Here's how the part is built. I have some questions about the finished solid (model axes, mm). Face numbers are marked on the shaded views. A direction names the side the tool comes from. Round coordinates to 2 decimals unless told otherwise and drop trailing zeros. Loops run counter-clockwise (first coordinate to the right, second up) from the corner with the lowest first, then second, coordinate; pieces in that order, holes last. Notation, with made-up numbers: M -36.5,76.5 L -17.5,76.5 A12 ccw -17.5,83.5 Z; hole C -9.75,52.25 d11. An arc over 180 degrees is marked long. Answer as CSV lines item,"result".
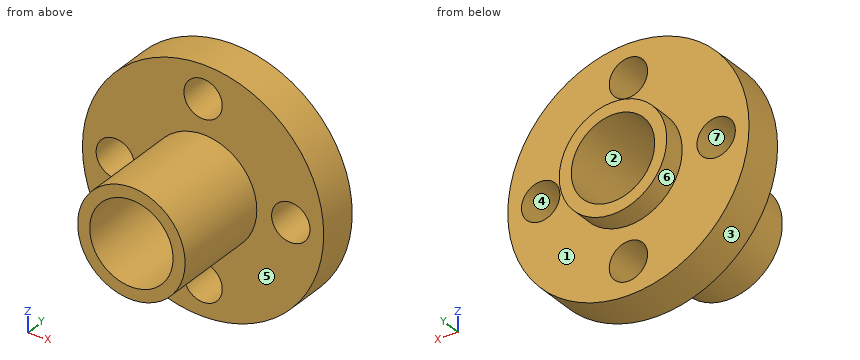
Autodesk Inventor part; units mm, degrees
ref_plane "YZ Plane" through (0, 0, 0) normal (1, 0, 0) x (0, 1, 0)
ref_plane "XZ Plane" through (0, 0, 0) normal (0, 1, 0) x (-1, 0, 0)
ref_plane "XY Plane" through (0, 0, 0) normal (0, 0, 1) x (1, 0, 0)
sketch "Sketch1" plane through (0, 0, 0) normal (0, 0, 1) x (1, 0, 0)
  line L0 (3.8, 0) -> (3.8, 15)
  line L1 (3.8, 15) -> (4.9, 15)
  line L2 (4.9, 15) -> (4.9, 13)
  line L3 (4.9, 13) -> (11, 13)
  line L4 (11, 13) -> (11, 9.3)
  line L5 (11, 9.3) -> (4.9, 9.3)
  line L6 (4.9, 9.3) -> (4.9, 0)
  line L7 (4.9, 0) -> (3.8, 0)
  line L8 (-2.2, 0) -> (13.2, 0)
  line L9 (0, -3) -> (0, 18)
  point P0 (0, 0)
  point P1 (4.35, 0)
  point P2 (4.35, 15)
  point P3 (11, 11.15)
  dimension "d0" = 3.7
  dimension "d1" = 15
  dimension "d2" = 2
  dimension "d3" = 11
  dimension "d4" = 6.1
  dimension "d5" = 3.8
revolve "Revolution1" add sketch "Sketch1" angle 360 about axis through (0, -10, 0) along (0, 1, 0)
sketch "Sketch2" plane through (0, 13, 0) normal (0, 1, 0) x (1, 0, 0)
  circle A0 centre (0, 8) radius 1.75
  point P0 (0, 0)
  dimension "d7" = 3.5
  dimension "d8" = 8
extrude "Extrusion1" cut sketch "Sketch2" against normal up to surface (3.7 mm away)
pattern_circular "Circular Pattern1" count 4 over 360 about axis through (0, 11.15, 0) along (0, 1, 0) of "Extrusion1"
properties part number "Lead nut"
1. I want a section at D-D, the plane y = 8. Please give me the cut outline in (x, z).
Evaluation:
outline,"C 0,0 d9.8; hole C 0,0 d7.6"
2. I want a section at A-A, the plane x = -8. Please give me the cut outline in (y, z), and give its area (3 significant figures).
Evaluation:
outline,"M 9.3,-7.55 L 13,-7.55 L 13,-1.75 L 9.3,-1.75 Z; M 9.3,1.75 L 13,1.75 L 13,7.55 L 9.3,7.55 Z"
area,"42.9 mm²"
3. I want a section at C-C, the plane z = 0. Please give me the cut outline in (x, y), and give its area (3 significant figures).
Evaluation:
outline,"M -11,9.3 L -9.75,9.3 L -9.75,13 L -11,13 Z; M -6.25,9.3 L -4.9,9.3 L -4.9,0 L -3.8,0 L -3.8,15 L -4.9,15 L -4.9,13 L -6.25,13 Z; M 3.8,0 L 4.9,0 L 4.9,9.3 L 6.25,9.3 L 6.25,13 L 4.9,13 L 4.9,15 L 3.8,15 Z; M 9.75,9.3 L 11,9.3 L 11,13 L 9.75,13 Z"
area,"52.2 mm²"
4. Which directions (+Z, -Z, +X, -X, +Y, -Y) give clear straight access to the entire face, cutting with the end or side of a thin tool? Please do the marked faces 5, 6 and 7.
Evaluation:
face 5,"-Y"
face 6,"+Y"
face 7,"+Y, -Y"
5. If I drill on line 1 (Z direction, x = 0, y = 12.25); line 2 (Y direction, x = -6.25, z = 3), over which ranges is the centre line in solid material (lowest first)? Write a range as [from, to].
Evaluation:
line 1,"z = [-11, -9.75], [-6.25, -3.8], [3.8, 6.25], [9.75, 11]"
line 2,"y = [9.3, 13]"
6. We'd pull the mould along Z, two halves only. Please class the marked faces 1, 2, 3 and 4: pulls with the +Z half, pulls with the -Z half, needs draft (parallel to the pull), parting line crosses it, or undercut.
Evaluation:
face 1,"needs draft"
face 2,"undercut"
face 3,"parting line crosses it"
face 4,"undercut"
7. For P1, Ø3, axis at y = 7.5, z = -2.5, coming from the -X side; P2, Ø4, axis at x = -7, z = -7, coming from the -Y side; P3, Ø3, axis at y = 11, z = 4.5, coming from the -X side, each with a flat end and sliding along its axis, tell me the tip position at first contact or that it passes through.
Evaluation:
P1,"stops at x = -4.8"
P2,"stops at y = 9.3"
P3,"stops at x = -10.58"
8. I want a section at B-B, the plane z = 8.75. Please give me the cut outline in (x, y).
Evaluation:
outline,"M -6.67,9.3 L -1.58,9.3 L -1.58,13 L -6.67,13 Z; M 1.58,9.3 L 6.67,9.3 L 6.67,13 L 1.58,13 Z"
